Read the model definition and answer for the solid it produces. Units are mm, in the model's axes. A direction names the side the tool comes from. Coordinates: 2 decimals unless noted, no trailing zeros. Order: outer loops, then holes, each group sorted by start corner. A loop starts at its lowest first (then second) coordinate and runs counter-clockwise, first axis right, second up. Notation, with made-up numbers: M 89.5,-4.5 L 116.5,-4.5 A15 ccw 116.5,-0.5 Z; hole C 37,61.25 d8. An arc over 180 degrees is marked long. One line per question, with ' | ' between items. Start each with the question number.
1) Consider probe 1 along Z at (x, y) = (86.5, 14); probe 2 along Y at (x, z) = (109.5, 50); probe 3 along X at (y, z) = (400, 119). Determine where each line is inside the solid, lowest interval first.
2) Find section B-B, the plane z = 56.5. Write down the section's boundary in (x, y).
3) The mould has two halves that part along Z. Classify faces 1 (the face through (39.152, 108.922, 100.933)), 2 (the face through (198, 54, -4)), 3 (the face through (200, -27, 1)), 4 (the face through (99, -2, -93.898)): +Z half, -Z half, draft (parallel to the pull), parting line (faces both ways), or undercut.
4) Find section C-C, the plane x = 13.5. Write down the section's boundary in (y, z), plus the area to 3 significant figures.
5) Given P1, Ø1, axis at x = 107.5, y = 66.5, coming from the +Z side; P2, Ø1, axis at x = 199, z = -26.5, coming from the +Y side, each flat-ended and moving along its own axis, determine where each tip first touches the part or whether it passes through.
6) Find section A-A, the plane y = 58. Write down the section's boundary in (x, z).
7) Find section D-D, the plane y = -41.5. Write down the section's boundary in (x, z), plus the area to 3 significant figures.
8) A tool of negligible diameter and unlimited length cuts with its end or side. For faces 5 (the face through (33, 749, 171.355)), 6 (the face through (31.561, 760.607, 154.799)), 7 (the face through (30.58, 428.68, 133.87)), from which of +Z, -Z, +X, -X, +Y, -Y can it reach the whole face along a straight path? Write none if from no direction.
from build123d import *

# Parameters (mm, degrees)
SKETCH1_W           = 187.796310486
SKETCH1_H           = 259.782504146
BOSS_EXTRUDE1_DEPTH = 200
SKETCH2_W           = 141.715117515
SKETCH2_H           = 96.14369286
CUT_EXTRUDE1_DEPTH  = 2
SKETCH3_R           = 11.367887844


with BuildPart() as part:
    # Sketch1 → Boss-Extrude1 (new body)
    with BuildSketch(Plane(origin=(0, 0, 0), x_dir=(0, 0, -1), z_dir=(1, 0, 0))):
        Rectangle(SKETCH1_W, SKETCH1_H)
    extrude(amount=BOSS_EXTRUDE1_DEPTH)

    # Sketch2 → Cut-Extrude1 (cut)
    with BuildSketch(Plane(origin=(200, 0, 0), x_dir=(0, 0, -1), z_dir=(1, 0, 0))):
        with Locations((5.289494402, 53.694775969)):
            Rectangle(SKETCH2_W, SKETCH2_H)
    extrude(amount=-CUT_EXTRUDE1_DEPTH, mode=Mode.SUBTRACT)

    # Sweep3: sweep along a curve in space
    with BuildLine() as sweep3_path:
        Line((33.040603642, 99.336066007, 93.898155243), (33.040603642, 99.336066007, 107.772716538))
        ThreePointArc((33.040603642, 114.336066007, 122.772716538), (33.040603642, 103.729464289, 118.379318255), (33.040603642, 99.336066007, 107.772716538))
        Line((33.040603642, 114.336066007, 122.772716538), (33.040603642, 734.336066007, 122.772716538))
        ThreePointArc((33.040603642, 734.336066007, 122.772716538), (33.040603642, 744.942667725, 127.16611482), (33.040603642, 749.336066007, 137.772716538))
        Line((33.040603642, 749.336066007, 137.772716538), (33.040603642, 749.336066007, 171.355386401))
    # Sketch3 → Sweep3 (sweep)
    with BuildSketch(Plane.XY.offset(93.898155243)):
        with Locations((33.040603642, 99.336066007)):
            Circle(SKETCH3_R)
    sweep(path=sweep3_path.line)


solid = part.part
Report:
1) probe 1: z = -93.9 to 93.9 | probe 2: y = -129.89 to 129.89 | probe 3: x = 22.32 to 43.76
2) outline: M 0,-129.89 L 200,-129.89 L 200,5.62 L 198,5.62 L 198,101.77 L 200,101.77 L 200,129.89 L 0,129.89 Z
3) face 1: undercut | face 2: undercut | face 3: draft | face 4: -Z half
4) outline: M -129.89,-93.9 L 129.89,-93.9 L 129.89,93.9 L -129.89,93.9 Z | area: 48,800 mm^2
5) P1: stops at z = 93.9 | P2: stops at y = 129.89
6) outline: M 0,-93.9 L 200,-93.9 L 200,-76.15 L 198,-76.15 L 198,65.57 L 200,65.57 L 200,93.9 L 0,93.9 Z
7) outline: M 0,-93.9 L 200,-93.9 L 200,93.9 L 0,93.9 Z | area: 37,600 mm^2
8) face 5: +Z, +X, -X, +Y, -Y | face 6: +Z | face 7: none
